```python
from build123d import *

# Parameters (mm, degrees)
SKETCH_1_W          = 10
SKETCH_1_H          = 10
SKETCH_1_W_2        = 8
SKETCH_1_H_2        = 8
EXTRUDE_1_DEPTH     = 700
SKETCH_2_R          = 2
CUT_EXTRUDE_1_DEPTH = 701.089280021


with BuildPart() as part:
    # ｽｹｯﾁ1 → 押し出し-薄板1 (new body)
    with BuildSketch(Plane(origin=(0, 0, 0), x_dir=(0, 0, -1), z_dir=(1, 0, 0))):
        Rectangle(SKETCH_1_W, SKETCH_1_H)
        Rectangle(SKETCH_1_W_2, SKETCH_1_H_2, mode=Mode.SUBTRACT)
    extrude(amount=EXTRUDE_1_DEPTH)

    # ｽｹｯﾁ2 → ｶｯﾄ - 押し出し1 (cut, through all)
    with BuildSketch(Plane(origin=(0, 5, 0), x_dir=(1, 0, 0), z_dir=(0, 1, 0))):
        with Locations(Location((695, 0, 0), (0, 0, 270))):
            Circle(SKETCH_2_R)
        with Locations(Location((5, 0, 0), (0, 0, 270))):
            Circle(SKETCH_2_R)
        with Locations(Location((501, 0, 0), (0, 0, 270))):
            Circle(SKETCH_2_R)
        with Locations(Location((199, 0, 0), (0, 0, 270))):
            Circle(SKETCH_2_R)
    extrude(amount=-CUT_EXTRUDE_1_DEPTH, mode=Mode.SUBTRACT)


solid = part.part
```
The listing builds one solid part. Answer for the finished solid, in the listing's coordinates (mm). Coordinates: 2 decimals unless noted, no trailing zeros. Write each loop counter-clockwise with the first axis right and the second up, starting at its lowest first coordinate (ties: lowest second). Pieces come first, ordered by that corner, then holes. Notation, with made-up numbers: (5.5, 21) - (47.5, 21) arc R35 ccw to (47.5, 55) - close; hole circle Ø6 at (11.25, 61). An arc over 180 degrees is marked (long way). Return JSON: item names as keys, results as strings. Group by question number.
1. A cutting plane is placed at C-C, the plane z = 0. Give the number of separate pieces and of enclosed holes in the cut face, plus the area to 3 significant figures.
2. A cutting plane is placed at B-B, the plane x = 332.5. Determine the outline of the cut face in (y, z), plus the area to 3 significant figures.
3. A cutting plane is placed at A-A, the plane y = 1.75. Determine the outline of the cut face in (x, z), plus the area to 3 significant figures.
4. Straight lines are drawn through the part: L1, parallel to X at y = -4.65, z = 0; L2, parallel to Y at x = 395.5, z = -3.25; L3, parallel to Z at x = 695, y = -4.3. For each, find the intervals that lie inside material, in ascending order.
Ans:
{
 "1": {"separate pieces": "10", "enclosed holes": "0", "area": "1,370 mm²"},
 "2": {"outline": "(-5, -5) - (5, -5) - (5, 5) - (-5, 5) - close; hole (-4, -4) - (4, -4) - (4, 4) - (-4, 4) - close", "area": "36.0 mm²"},
 "3": {"outline": "(0, -5) - (700, -5) - (700, -4) - (0, -4) - close; (0, 4) - (700, 4) - (700, 5) - (0, 5) - close", "area": "1,400 mm²"},
 "4": {"L1": "0 to 3, 7 to 197, 201 to 499, 503 to 693, 697 to 700", "L2": "-5 to -4, 4 to 5", "L3": "-5 to -2, 2 to 5"}
}
